from build123d import *

# Parameters (mm, degrees)
F0_W     = 20
F0_H     = 25
F0_R     = 6.5
F0_R_2   = 2.5
F0_H_2   = 2
F1_DEPTH = 5
F2_DEPTH = 45
F3_START = 20
F3_DEPTH = 5
F4_START = 40
F4_DEPTH = 5
F6_D     = 5
F6_DEPTH = 12.7
F6_TIP   = 1.5021515476


with BuildPart() as f1:
    # F0 (on Top) → F1 (new body)
    with BuildSketch(Plane.XY):
        Rectangle(F0_W, F0_H)
        Circle(F0_R, mode=Mode.SUBTRACT)
        Circle(F0_R)
        Circle(F0_R_2, mode=Mode.SUBTRACT)
        with Locations((0, 13.5)):
            Rectangle(F0_W, F0_H_2)
        with Locations((0, -25)):
            Rectangle(F0_W, F0_H)
        with Locations((0, -25)):
            Circle(F0_R, mode=Mode.SUBTRACT)
        with Locations((0, -25)):
            Circle(F0_R)
        with Locations((0, -25)):
            Circle(F0_R_2, mode=Mode.SUBTRACT)
        Polygon((12, -12.5), (10, -12.5), (10, -37.5), (10, -39.5), (12, -39.5), align=None)
        with Locations((0, -38.5)):
            Rectangle(F0_W, F0_H_2)
        Polygon((10, 14.5), (10, 12.5), (10, -12.5), (12, -12.5), (12, 14.5), align=None)
    extrude(amount=F1_DEPTH)

    # F0 (on Top) → F2 (join)
    with BuildSketch(Plane.XY):
        Polygon((12, -12.5), (10, -12.5), (10, -37.5), (10, -39.5), (12, -39.5), align=None)
        Polygon((10, 14.5), (10, 12.5), (10, -12.5), (12, -12.5), (12, 14.5), align=None)
    extrude(amount=F2_DEPTH)

    # F0 (on Top) → F3 (join)
    with BuildSketch(Plane.XY.offset(F3_START)):
        Rectangle(F0_W, F0_H)
        Circle(F0_R, mode=Mode.SUBTRACT)
        Circle(F0_R)
        Circle(F0_R_2, mode=Mode.SUBTRACT)
        with Locations((0, 13.5)):
            Rectangle(F0_W, F0_H_2)
        Polygon((12, -12.5), (10, -12.5), (10, -37.5), (10, -39.5), (12, -39.5), align=None)
        with Locations((0, -25)):
            Rectangle(F0_W, F0_H)
        with Locations((0, -25)):
            Circle(F0_R, mode=Mode.SUBTRACT)
        with Locations((0, -25)):
            Circle(F0_R)
        with Locations((0, -25)):
            Circle(F0_R_2, mode=Mode.SUBTRACT)
        with Locations((0, -38.5)):
            Rectangle(F0_W, F0_H_2)
        Polygon((10, 14.5), (10, 12.5), (10, -12.5), (12, -12.5), (12, 14.5), align=None)
    extrude(amount=F3_DEPTH)

    # F0 (on Top) → F4 (join)
    with BuildSketch(Plane.XY.offset(F4_START)):
        with Locations((0, 13.5)):
            Rectangle(F0_W, F0_H_2)
        Rectangle(F0_W, F0_H)
        Circle(F0_R, mode=Mode.SUBTRACT)
        Circle(F0_R)
        Circle(F0_R_2, mode=Mode.SUBTRACT)
        with Locations((0, -25)):
            Rectangle(F0_W, F0_H)
        with Locations((0, -25)):
            Circle(F0_R, mode=Mode.SUBTRACT)
        with Locations((0, -25)):
            Circle(F0_R)
        with Locations((0, -25)):
            Circle(F0_R_2, mode=Mode.SUBTRACT)
        Polygon((12, -12.5), (10, -12.5), (10, -37.5), (10, -39.5), (12, -39.5), align=None)
        with Locations((0, -38.5)):
            Rectangle(F0_W, F0_H_2)
        Polygon((10, 14.5), (10, 12.5), (10, -12.5), (12, -12.5), (12, 14.5), align=None)
    extrude(amount=F4_DEPTH)

    # F6
    with Locations(Plane(origin=(10, 0, 0), x_dir=(0, -1, 0), z_dir=(-1, 0, 0))):
        with Locations((0, 30), (20, 30)):
            Hole(F6_D / 2, depth=F6_DEPTH)
            with Locations((0, 0, -(F6_DEPTH + F6_TIP / 2))):  # 118° drill point
                Cone(0, F6_D / 2, F6_TIP, mode=Mode.SUBTRACT)


solid = f1.part
Design review of the part built by this model. Coordinates are the model's own, in mm. A direction names the side the tool comes from. Round coordinates to 2 decimals unless told otherwise and drop trailing zeros. Order: outer loops, then holes, each group sorted by start corner. A loop starts at its lowest first (then second) coordinate and runs counter-clockwise, first axis right, second up. Notation, with made-up numbers: M -36,34 L 20,34 A19 ccw 20,49 Z; hole C 66,66 d10. An arc over 180 degrees is marked long. Answer as CSV lines item,"result". Start each with the question number.
1) Tool access review of faces 4 (the face through (10, -12, 12)), 5 (the face through (11.01, 1.34, 32.11)): name each direction out of +Z, -Z, +X, -X, +Y, -Y from which nothing blocks a thin tool from reaching the whole face with its end or side.
2) The part is to be moulded in two halves that separate along X. For faces 1 (the face through (0, -12, 25)), 2 (the face through (-0.33, -22.52, 2.46)), 3 (the face through (10, -12, 32)), say which applies: +X half, -X half, draft (parallel to the pull), parting line (faces both ways), or undercut.
3) Add section C-C (y = -20). Give the boundary of the cut face in (x, z), then the cut area to 3 significant figures.
4) Wall thickness on line 1 along Z through (x, y) = (5.5, -2); line 2 along Y through (x, z) = (0, 3); line 3 along X through (y, z) = (-35, 17.5): over which ranges is each line inside the solid? List them lowest first. Write a range as [from, to].
5) Add section B-B (z = 30). Give the boundary of the cut face in (x, y).
6) Add section A-A (x = 5.5). Give the boundary of the cut face in (y, z).
7) Add section D-D (y = -34). Give the boundary of the cut face in (x, z).
Resolved:
1,face 4,"-X, +Y, -Y"
1,face 5,"+X, -X"
2,face 1,"draft"
2,face 2,"undercut"
2,face 3,"-X half"
3,outline,"M -10,0 L 12,0 L 12,27.5 L 10,27.5 L 10,25 L -10,25 L -10,20 L 10,20 L 10,5 L -10,5 Z; M -10,40 L 10,40 L 10,32.5 L 12,32.5 L 12,45 L -10,45 Z"
3,area,"380 mm^2"
4,line 1,"[0, 5], [20, 25], [40, 45]"
4,line 2,"[-39.5, -27.5], [-22.5, -2.5], [2.5, 14.5]"
4,line 3,"[10, 12]"
5,outline,"M 10,-39.5 L 12,-39.5 L 12,-22.5 L 10,-22.5 Z; M 10,-17.5 L 12,-17.5 L 12,-2.5 L 10,-2.5 Z; M 10,2.5 L 12,2.5 L 12,14.5 L 10,14.5 Z"
6,outline,"M -39.5,0 L 14.5,0 L 14.5,5 L -39.5,5 Z; M -39.5,20 L 14.5,20 L 14.5,25 L -39.5,25 Z; M -39.5,40 L 14.5,40 L 14.5,45 L -39.5,45 Z"
7,outline,"M -10,0 L 12,0 L 12,45 L -10,45 L -10,40 L 10,40 L 10,25 L -10,25 L -10,20 L 10,20 L 10,5 L -10,5 Z"
